from build123d import *

# Parameters (mm, degrees)
EXTRUDE_1_DEPTH = 55
CHAMFER_1_SIZE  = 0.5


with BuildPart() as part:
    # 草图1 → 凸台-拉伸1 (new body)
    with BuildSketch(Plane(origin=(0, 0, 0), x_dir=(0, 0, -1), z_dir=(1, 0, 0))):
        Polygon((0, 6), (0, 0), (5.638155725, -2.05212086), (5.638155725, 6), align=None)
    extrude(amount=EXTRUDE_1_DEPTH)

    # 倒角1
    chamfer_1_edges = [part.edges().sort_by_distance(p)[0] for p in [
        (27.5, 6, -5.638155725),
    ]]
    chamfer(chamfer_1_edges, length=CHAMFER_1_SIZE)


solid = part.part
The listing builds one solid part. Answer for the finished solid, in the listing's coordinates (mm). Coordinates: 2 decimals unless noted, no trailing zeros. Loops run counter-clockwise (first coordinate to the right, second up) from the corner with the lowest first, then second, coordinate; pieces in that order, holes last. Notation, with made-up numbers: (40, 63) -> (93, 63) arc R16 cw to (93, 86) -> close; hole circle Ø9 at (38, 81.25). An arc over 180 degrees is marked (long way). Write item = value, one per line. Start each with the question number.
1) A cutting plane is placed at C-C (z = -1.2). Give the vertices of the cut face in (x, y), then the cut area to 3 significant figures.
2) A cutting plane is placed at A-A (x = 19). Give the vertices of the cut face in (y, z).
3) A cutting plane is placed at B-B (y = -1.5). Give the vertices of the cut face in (x, z), then the cut area to 3 significant figures.
4) Straight lines are drawn through the part: line 1 (Y direction, x = 50, z = -2.45); line 2 (Y direction, x = 35.5, z = -0.55); line 3 (Z direction, x = 26, y = 5.75). For each, find the intervals that lie inside material, in ascending order. Write a range as from..to.
Responses:
q1.outline = (0, -0.44) -> (55, -0.44) -> (55, 6) -> (0, 6) -> close
q1.area = 354 mm²
q2.outline = (-2.05, -5.64) -> (5.5, -5.64) -> (6, -5.14) -> (6, 0) -> (0, 0) -> close
q3.outline = (0, -5.64) -> (55, -5.64) -> (55, -4.12) -> (0, -4.12) -> close
q3.area = 83.4 mm²
q4.line_1 = -0.89..6
q4.line_2 = -0.2..6
q4.line_3 = -5.39..0
